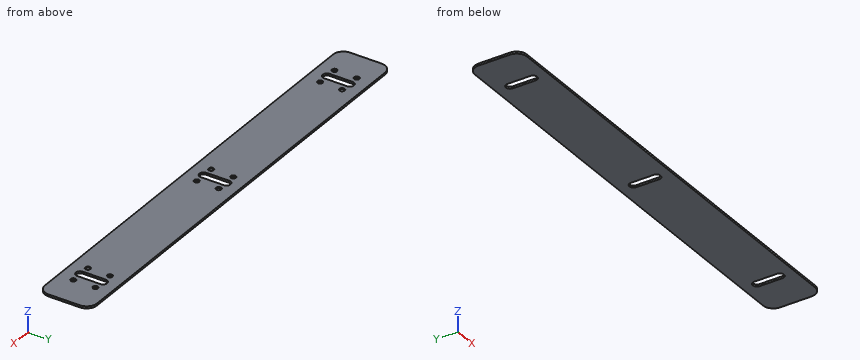
from build123d import *

# Parameters (mm, degrees)
BOSS_EXTRUDE1_DEPTH = 0.2
SKETCH2_R           = 0.25
CUT_EXTRUDE1_DEPTH  = 0.1


with BuildPart() as part:
    # Sketch1 → Boss-Extrude1 (new body)
    with BuildSketch(Plane.XY):
        with BuildLine():
            Line((-13.983305509, 11.944444444), (28.016694491, 11.944444444))
            ThreePointArc((28.016694491, 11.944444444), (28.723801272, 11.651551226), (29.016694491, 10.944444444))
            Line((29.016694491, 10.944444444), (29.016694491, 7.944444444))
            ThreePointArc((29.016694491, 7.944444444), (28.723801272, 7.237337663), (28.016694491, 6.944444444))
            Line((28.016694491, 6.944444444), (-13.983305509, 6.944444444))
            ThreePointArc((-13.983305509, 6.944444444), (-14.69041229, 7.237337663), (-14.983305509, 7.944444444))
            Line((-14.983305509, 7.944444444), (-14.983305509, 10.944444444))
            ThreePointArc((-14.983305509, 10.944444444), (-14.69041229, 11.651551226), (-13.983305509, 11.944444444))
        make_face()
        with BuildLine():
            Line((-10.583305509, 10.544444444), (-10.583305509, 8.344444444))
            ThreePointArc((-10.583305509, 8.344444444), (-10.983305509, 7.944444444), (-11.383305509, 8.344444444))
            Line((-11.383305509, 8.344444444), (-11.383305509, 10.544444444))
            ThreePointArc((-11.383305509, 10.544444444), (-10.983305509, 10.944444444), (-10.583305509, 10.544444444))
        make_face(mode=Mode.SUBTRACT)
        with BuildLine():
            Line((7.416694491, 10.544444444), (7.416694491, 8.344444444))
            ThreePointArc((7.416694491, 8.344444444), (7.016694491, 7.944444444), (6.616694491, 8.344444444))
            Line((6.616694491, 8.344444444), (6.616694491, 10.544444444))
            ThreePointArc((6.616694491, 10.544444444), (7.016694491, 10.944444444), (7.416694491, 10.544444444))
        make_face(mode=Mode.SUBTRACT)
        with BuildLine():
            Line((25.416694491, 10.544444444), (25.416694491, 8.344444444))
            ThreePointArc((25.416694491, 8.344444444), (25.016694491, 7.944444444), (24.616694491, 8.344444444))
            Line((24.616694491, 8.344444444), (24.616694491, 10.544444444))
            ThreePointArc((24.616694491, 10.544444444), (25.016694491, 10.944444444), (25.416694491, 10.544444444))
        make_face(mode=Mode.SUBTRACT)
    extrude(amount=BOSS_EXTRUDE1_DEPTH)

    # Sketch2 → Cut-Extrude1 (cut)
    with BuildSketch(Plane.XY.offset(0.2)):
        with Locations((-9.922645337, 10.505104616)):
            Circle(SKETCH2_R)
        with Locations((-9.922645337, 8.383784273)):
            Circle(SKETCH2_R)
        with Locations((-12.043965681, 8.383784273)):
            Circle(SKETCH2_R)
        with Locations((-12.043965681, 10.505104616)):
            Circle(SKETCH2_R)
        with Locations((8.077354663, 10.505104616)):
            Circle(SKETCH2_R)
        with Locations((5.956034319, 10.505104616)):
            Circle(SKETCH2_R)
        with Locations((5.956034319, 8.383784273)):
            Circle(SKETCH2_R)
        with Locations((8.077354663, 8.383784273)):
            Circle(SKETCH2_R)
        with Locations((26.077354663, 10.505104616)):
            Circle(SKETCH2_R)
        with Locations((23.956034319, 10.505104616)):
            Circle(SKETCH2_R)
        with Locations((23.956034319, 8.383784273)):
            Circle(SKETCH2_R)
        with Locations((26.077354663, 8.383784273)):
            Circle(SKETCH2_R)
    extrude(amount=-CUT_EXTRUDE1_DEPTH, mode=Mode.SUBTRACT)


solid = part.part
Design review of the part built by this model. Coordinates are the model's own, in mm. Give positions to 0.01 mm unless a question says otherwise; leave off trailing zeros. Loops run counter-clockwise (first coordinate to the right, second up) from the corner with the lowest first, then second, coordinate; pieces in that order, holes last. Notation, with made-up numbers: (-20.5, 42) -> (16.5, 42) arc R26 cw to (16.5, 75) -> close; hole circle Ø1 at (29, 12.25). An arc over 180 degrees is marked (long way). One line per question, with ' | ' between items. Start each with the question number.
(1) We need section B-B (z = 0.05). State the section outline as (x, y) points.
(2) For line 1 (X direction, y = 8.9, z = 0.15); line 2 (Y direction, x = 25, z = 0.15); line 3 (X direction, y = 11.6, z = 0.1), list the stretches that pass through material, from the lowest coordinate up.
(3) We need section A-A (y = 9.7). State the section outline as (x, z) points.
(4) Insertion check: P1, Ø0.6, axis at x = 24, y = 10.5, coming from the +Z side. The pin has a flat end and moves straight along its axis. Give the tip position at first contact, or say it passes through.
The answers:
1) outline: (-14.98, 7.94) arc R1 ccw to (-13.98, 6.94) -> (28.02, 6.94) arc R1 ccw to (29.02, 7.94) -> (29.02, 10.94) arc R1 ccw to (28.02, 11.94) -> (-13.98, 11.94) arc R1 ccw to (-14.98, 10.94) -> close; hole (-11.38, 8.34) arc R0.4 ccw to (-10.58, 8.34) -> (-10.58, 10.54) arc R0.4 ccw to (-11.38, 10.54) -> close; hole (6.62, 8.34) arc R0.4 ccw to (7.42, 8.34) -> (7.42, 10.54) arc R0.4 ccw to (6.62, 10.54) -> close; hole (24.62, 8.34) arc R0.4 ccw to (25.42, 8.34) -> (25.42, 10.54) arc R0.4 ccw to (24.62, 10.54) -> close
2) line 1: x = -14.98 to -11.38, -10.58 to 6.62, 7.42 to 24.62, 25.42 to 29.02 | line 2: y = 6.94 to 7.94, 10.94 to 11.94 | line 3: x = -14.74 to 28.77
3) outline: (-14.98, 0) -> (-11.38, 0) -> (-11.38, 0.2) -> (-14.98, 0.2) -> close; (-10.58, 0) -> (6.62, 0) -> (6.62, 0.2) -> (-10.58, 0.2) -> close; (7.42, 0) -> (24.62, 0) -> (24.62, 0.2) -> (7.42, 0.2) -> close; (25.42, 0) -> (29.02, 0) -> (29.02, 0.2) -> (25.42, 0.2) -> close
4) P1: stops at z = 0.2
